The listing builds one solid part. Answer for the finished solid, in the listing's coordinates (mm). Give positions to 0.01 mm unless a question says otherwise; leave off trailing zeros. Write each loop counter-clockwise with the first axis right and the second up, starting at its lowest first coordinate (ties: lowest second). Pieces come first, ordered by that corner, then holes.
```python
from build123d import *

# Parameters (mm, degrees)
F1_DEPTH = 196.85
F2_SIZE2 = 18.25624
F2_SIZE  = 18.25624
F3_SIZE  = 18.25624


# Not quite as in the source:
# - a fillet or chamfer is up to 0.001 mm smaller than in the source, because OpenCascade refuses the exact size


with BuildPart() as f1:
    # F0 (on Top) → F1 (new body, symmetric)
    with BuildSketch(Plane.XY):
        Polygon((9.128125, -98.425), (9.128125, 114.3), (-9.128125, 114.3), (-9.128125, -114.3), (9.128125, -114.3), (9.128125, -104.775), (2.778125, -104.775), (2.778125, -98.425), align=None)
    extrude(amount=F1_DEPTH, both=True)

    # F2 (size 18.25625 and 18.25625 in the source; OpenCascade refuses exactly that, so slightly less here)
    f2_edges = [f1.edges().sort_by_distance(p)[0] for p in [
        (9.128125, 7.9375, 196.85),
    ]]
    chamfer(f2_edges, length=F2_SIZE, length2=F2_SIZE2)

    # F3 (size 18.25625 in the source; OpenCascade refuses exactly that, so slightly less here)
    f3_edges = [f1.edges().sort_by_distance(p)[0] for p in [
        (9.128125, 7.9375, -196.85),
    ]]
    chamfer(f3_edges, length=F3_SIZE)


solid = f1.part
```
Item 1: Consider probe 1 along Y at (x, z) = (7.5, -120.5) (3 decimals); probe 2 along Z at (x, y) = (-3.25, 27); probe 3 along Z at (x, y) = (3.5, -84.5). Determine where each line is inside the solid, lowest interval first.
Conclusion:
probe 1: y = -114.3 to -104.775, -98.425 to 114.3
probe 2: z = -190.97 to 190.97
probe 3: z = -184.22 to 184.22
Item 2: This flat-tipped pin is pushed along its axis until it touches: P1, Ø1.9, axis at y = -103, z = 26.5, coming from the +X side. Where does it stop, or does it pass through?
Conclusion:
P1: stops at x = 2.78
Item 3: A cutting plane is placed at B-B, the plane x = -3. Give the vertices of the cut face in (y, z).
Conclusion:
outline: (-114.3, -190.72) - (114.3, -190.72) - (114.3, 190.72) - (-114.3, 190.72) - close
